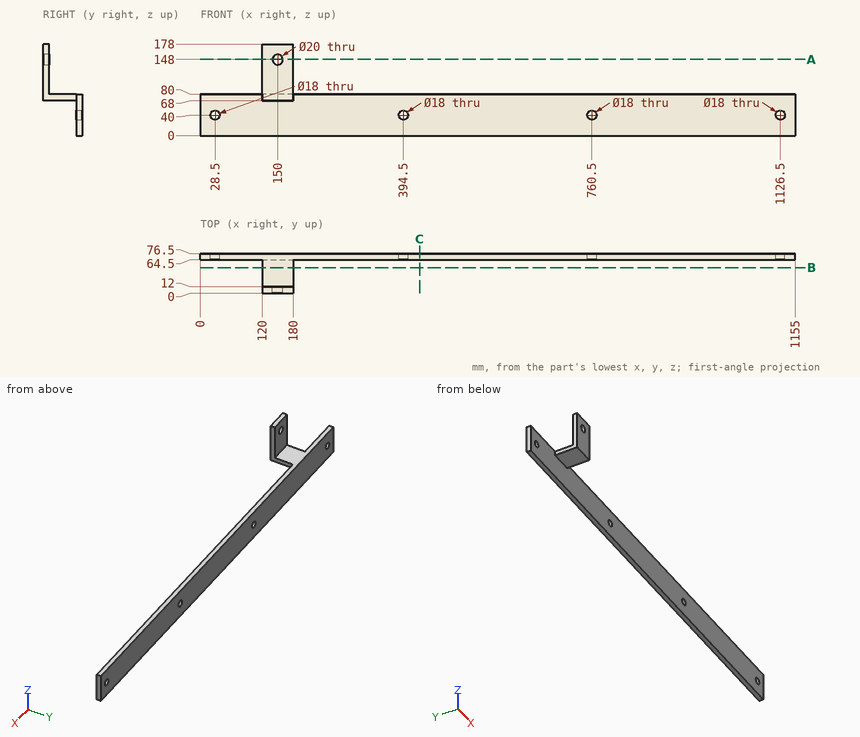
Drawing for the job (mm, zero at the part's lowest x, y, z). Give positions to 0.01 mm unless a question says otherwise; leave off trailing zeros. Order: outer loops, then holes, each group sorted by start corner. A loop starts at its lowest first (then second) coordinate and runs counter-clockwise, first axis right, second up. Notation, with made-up numbers: M 41.5,39.25 L 48.5,39.25 A20 cw 48.5,60.25 Z; hole C 65,67 d11. An arc over 180 degrees is marked long. Write item = value, one per line. Start each with the question number.
(1) Slice it at B-B on y = 49.5. Write the cut outline in (x, z), plus the area to 3 significant figures.
(2) Probe L1, parallel to X at y = 72, z = 40; L2, parallel to Z at x = 150, y = 9.5; L3, parallel to Z at x = 28, y = 67. List the from-to ranges inside material, lowest first. Write a range as [from, to].
(3) Pin check, flat tips, straight feed: pin 1 Ø20.5 at (x, z) = (394.5, 40) entering from +Y; pin 2 Ø19.5 at (y, z) = (20.5, 127) entering from -X; pin 3 Ø16 at (x, z) = (760.5, 40) entering from +Y; pin 4 Ø18 at (x, y) = (142, 23.5) entering from -Z. Stop position of each tip, or through.
(4) Slice it at A-A on z = 148. Write the cut outline in (x, y).
(5) Slice it at C-C on x = 426. Write the cut outline in (y, z), plus the area to 3 significant figures.
Responses:
q1.outline = M 120,68 L 180,68 L 180,80 L 120,80 Z
q1.area = 720 mm2
q2.L1 = [0, 19.5], [37.5, 385.5], [403.5, 751.5], [769.5, 1117.5], [1135.5, 1155]
q2.L2 = [68, 138], [158, 178]
q2.L3 = [0, 31.01], [48.99, 80]
q3.pin_1 = 76.5
q3.pin_2 = 120
q3.pin_3 = through
q3.pin_4 = 68
q4.outline = M 120,0 L 140,0 L 140,12 L 120,12 Z; M 160,0 L 180,0 L 180,12 L 160,12 Z
q5.outline = M 64.5,0 L 76.5,0 L 76.5,80 L 64.5,80 Z
q5.area = 960 mm2
